Verification items for the finished model (mm, model axes). A direction names the side the tool comes from. Round coordinates to 2 decimals unless told otherwise and drop trailing zeros. Write each loop counter-clockwise with the first axis right and the second up, starting at its lowest first coordinate (ties: lowest second). Pieces come first, ordered by that corner, then holes. Notation, with made-up numbers: (2.5, 79.5) - (37.5, 79.5) arc R34 ccw to (37.5, 110.5) - close; hole circle Ø10 at (-14.75, 12). An arc over 180 degrees is marked (long way). Answer as a JSON object with one key per item and string values.
```python
from build123d import *

# Parameters (mm, degrees)
SALIENTE_EXTRUIR1_DEPTH = 325
VACIADO1_T              = -3
CROQUIS2_W              = 76.381162613
CROQUIS2_H              = 128.156475552
CORTAR_EXTRUIR1_DEPTH   = 697.992520796


with BuildPart() as part:
    # Croquis1 → Saliente-Extruir1 (new, symmetric)
    with BuildSketch(Plane.XY):
        Polygon((0, 0), (0, 120), (600, 120), (705.985097206, 60), (705.985097206, 0), align=None)
    extrude(amount=SALIENTE_EXTRUIR1_DEPTH, both=True)

    # Vaciado1
    vaciado1_openings = [part.faces().sort_by_distance(p)[0] for p in [
        (352.992548603, 0, 0),
    ]]
    offset(amount=VACIADO1_T, openings=vaciado1_openings, kind=Kind.INTERSECTION)

    # Croquis2 → Cortar-Extruir1 (cut, through all)
    with BuildSketch(Plane(origin=(197.068972386, 348.106236577, 0), x_dir=(0.8702271613704161, -0.4926506750357577, 0), z_dir=(0.4926506750357577, 0.8702271613704161, 0))):
        with Locations((523.913291213, 0)):
            Rectangle(CROQUIS2_W, CROQUIS2_H)
    extrude(amount=-CORTAR_EXTRUIR1_DEPTH, mode=Mode.SUBTRACT)


solid = part.part
```
Q1. Material ranges on line 1 along X through (y, z) = (18, -83); line 2 along Z through (x, y) = (593.5, 86); line 3 along Y through (x, z) = (472.5, 200.5), recorded low to high. Write a range as [from, to].
Geometry check:
{"line 1": "x = [0, 3], [702.99, 705.99]", "line 2": "z = [-325, -322], [322, 325]", "line 3": "y = [117, 120]"}
Q2. Section check D-D, the plane z = -285. Record the cut outline in (x, y), then the cut area to 3 significant figures.
Geometry check:
{"outline": "(0, 0) - (3, 0) - (3, 117) - (599.21, 117) - (702.99, 58.25) - (702.99, 0) - (705.99, 0) - (705.99, 60) - (600, 120) - (0, 120) - close", "area": "2,690 mm2"}
Q3. Section check C-C, the plane x = 395.5. Record the cut outline in (y, z), then the cut area to 3 significant figures.
Geometry check:
{"outline": "(0, -325) - (120, -325) - (120, 325) - (0, 325) - (0, 322) - (117, 322) - (117, -322) - (0, -322) - close", "area": "2,650 mm2"}
Q4. Section check B-B, the plane z = 15.5. Record the cut outline in (x, y).
Geometry check:
{"outline": "(0, 0) - (3, 0) - (3, 117) - (599.21, 117) - (618.28, 106.2) - (619.76, 108.81) - (600, 120) - (0, 120) - close; (684.75, 68.57) - (702.99, 58.25) - (702.99, 0) - (705.99, 0) - (705.99, 60) - (686.23, 71.19) - close"}
Q5. Set-up check for faces 4 (the flat face through (358, 59, -322)), 5 (the flat face through (296, 120, 5)): record each of +Z, -Z, +X, -X, +Y, -Y from which the full face is reachable in a straight line by a thin tool's end or side.
Geometry check:
{"face 4": "-Y", "face 5": "+Z, -Z, +X, -X, +Y"}
Q6. Section check A-A, the plane y = 20. Record the cut outline in (x, z), then the cut area to 3 significant figures.
Geometry check:
{"outline": "(0, -325) - (705.99, -325) - (705.99, 325) - (0, 325) - close; hole (3, -322) - (702.99, -322) - (702.99, 322) - (3, 322) - close", "area": "8,100 mm2"}
Q7. Release check for a two-part mould opening along X. For faces 1 (the flat face through (358, 61, 325)), 2 (the flat face through (616.92, 110.42, 4.55)), 3 (the flat face through (358, 59, 322)) record: released by +X, released by -X, zero draft, split by the parting line, or undercut.
Geometry check:
{"face 1": "zero draft", "face 2": "released by +X", "face 3": "undercut"}
Q8. Gauge pin test, flat ends, axial feed: P1, Ø12, axis at x = 73.5, z = 191.5, coming from the -Y side; P2, Ø20, axis at x = 663.5, y = 93, coming from the -Z side. Record the tip position at first contact, or that the pin passes through.
Geometry check:
{"P1": "stops at y = 117", "P2": "stops at z = -325"}
